from build123d import *

# Parameters (mm, degrees)
F0_R           = 9.656937
F1_DEPTH       = 5.334
F2_R           = 5.306447
F3_DEPTH       = 5.588
F5_D           = 6.858
F5_CSINK_D     = 13.716
F5_CSINK_ANGLE = 82


with BuildPart() as f1:
    # F0 (on Top) → F1 (new body)
    with BuildSketch(Plane.XY):
        Circle(F0_R)
    extrude(amount=F1_DEPTH)

    # F2 (on face) → F3 (join)
    with BuildSketch(Plane.XY.offset(5.334)):
        Circle(F2_R)
    extrude(amount=F3_DEPTH)

    # F5 (through all)
    with Locations(Plane(origin=(0, 0, 0), x_dir=(1, 0, 0), z_dir=(0, 0, -1))):
        with Locations((0, 0)):
            CounterSinkHole(F5_D / 2, F5_CSINK_D / 2, counter_sink_angle=F5_CSINK_ANGLE)


solid = f1.part
Could you check a few things on this model? Use its own coordinates, in mm. A direction names the side the tool comes from. Round coordinates to 2 decimals unless told otherwise and drop trailing zeros. Write each loop counter-clockwise with the first axis right and the second up, starting at its lowest first coordinate (ties: lowest second). Pieces come first, ordered by that corner, then holes. Notation, with made-up numbers: (-23.5, -16) - (16.5, -16) arc R8 cw to (16.5, -6) - close; hole circle Ø7 at (3, -35). An arc over 180 degrees is marked (long way). Put each result on its own line as item: value. Start each with the question number.
(1) For faces 1 (the cylindrical face through (5.061, 1.594, 8.089)), 2 (the flat face through (-7, -2, 0)), which set-ups out of +Z, -Z, +X, -X, +Y, -Y let a thin tool reach every point of the face, with its end or its side?
(2) I want a section at A-A, the plane x = 0. Please give me the cut outline in (y, z).
(3) I want a section at D-D, the plane y = -7.5. Please give me the cut outline in (x, z).
(4) Thinking about a two-plate mould opening in X: for faces 3 (the conical face through (-3.43, -1.08, 3.75)), 4 (the cylindrical face through (4.456, -8.567, 2.63)), 5 (the flat face through (4, -4, 5.334)), 6 (the cylindrical face through (0.74, 3.35, 7.48)), which applies, released by +X, released by -X, zero draft, split by the parting line, or undercut?
(5) I need wall thicknesses on probe 1 along Y at (x, z) = (0, 8); probe 2 along Z at (x, y) = (-8.25, 2); probe 3 along Y at (x, z) = (-3.25, 1.25). Which ranges of each line are inside material? Lowest first, please.
(6) I want a section at C-C, the plane z = 3.25. Please give me the cut outline in (x, y), plus the area to 3 significant figures.
(7) Will these pins go through, and if not, where does the flat tip stop? pin 1 (6 mm diameter, centred on x = -1, y = -2.5, fed in from -Z); pin 2 (3 mm diameter, centred on x = 3.5, y = -3, fed in from -Z); pin 3 (1 mm diameter, centred on y = 7.5, z = 6.5, fed in from +X); pin 4 (6 mm diameter, centred on y = 3.5, z = 3, fed in from +X).
Here are the results:
1. face 1: +Z
1. face 2: -Z, +X, -X, +Y, -Y
2. outline: (-9.66, 0) - (-6.86, 0) - (-3.43, 3.94) - (-3.43, 10.92) - (-5.31, 10.92) - (-5.31, 5.33) - (-9.66, 5.33) - close; (3.43, 3.94) - (6.86, 0) - (9.66, 0) - (9.66, 5.33) - (5.31, 5.33) - (5.31, 10.92) - (3.43, 10.92) - close
3. outline: (-6.08, 0) - (6.08, 0) - (6.08, 5.33) - (-6.08, 5.33) - close
4. face 3: undercut
4. face 4: split by the parting line
4. face 5: zero draft
4. face 6: undercut
5. probe 1: y = -5.31 to -3.43, 3.43 to 5.31
5. probe 2: z = 0 to 5.33
5. probe 3: y = -9.09 to -4.77, 4.77 to 9.09
6. outline: circle Ø19.31 at (0, 0); hole circle Ø8.07 at (0, 0)
6. area: 242 mm^2
7. pin 1: stops at z = 1.34
7. pin 2: stops at z = 0.86
7. pin 3: passes through
7. pin 4: stops at x = 9.64
